Geometry check sheet. Reference: the model listing, model coordinates, mm. A direction names the side the tool comes from. Give positions to 0.01 mm unless a question says otherwise; leave off trailing zeros. Write each loop counter-clockwise with the first axis right and the second up, starting at its lowest first coordinate (ties: lowest second). Pieces come first, ordered by that corner, then holes. Notation, with made-up numbers: (64, 68) -> (76, 68) arc R15 ccw to (76, 88) -> close; hole circle Ø11 at (41, 63.5). An arc over 180 degrees is marked (long way). Write item = value, one per line. Start each with the question number.
1. Set-up check for faces 1 (the flat face through (-0.1, -7.3, -9)), 2 (the flat face through (3, 6, -11)), 3 (the flat face through (-6, 4, -9)): record each of +Z, -Z, +X, -X, +Y, -Y from which the full face is reachable in a straight line by a thin tool's end or side.
2. Mould release check, pull along Z, two halves, no side actions. Record for faces 4 (the flat face through (6, -4, -9)), 5 (the cylindrical face through (-7.25, 2.28, 1.17)), 6 (the flat face through (3, -6, 0)): pulls with the +Z half, pulls with the -Z half, needs draft (parallel to the pull), parting line crosses it, or undercut.
3. Thickness scan on line 1 along Z through (x, y) = (6.75, 2); line 2 along Z through (x, y) = (0.25, 0.75); line 3 along Z through (x, y) = (-0.75, 4.75). Record the ranges inside material, lowest first.
4. Depth check by flat-ended pin: P1, Ø1.5, axis at x = 0.5, z = -12.5, coming from the -Y side; P2, Ø3, axis at x = -6, y = 5, coming from the -Z side; P3, Ø3, axis at y = 6, z = -14.5, coming from the -X side. Enter the tip coordinate at first touch or a pass-through.
5. Cross-section at C-C, the plane z = -3.75. Record the cut outline in (x, y), plus the area to 3 significant figures.
6. Cross-section at A-A, the plane z = -19. Record the cut outline in (x, y), plus the area to 3 significant figures.
```python
from build123d import *

# Parameters (mm, degrees)
BOSS_EXTRUDE1_DEPTH        = 2
SKETCH3_R                  = 6.35
BOSS_EXTRUDE2_DEPTH        = 0.7
SKETCH4_R                  = 6.35
BOSS_EXTRUDE3_DEPTH        = 0.490747729
BOSS_EXTRUDE3_TAPER        = 60.000000001
SKETCH5_R                  = 5.5
BOSS_EXTRUDE4_DEPTH        = 6.309252271
BOSS_EXTRUDE5_DEPTH        = 5
CUT_EXTRUDE1_DEPTH         = 29.154677259
BOSS_EXTRUDE6_DEPTH        = 5
CUT_EXTRUDE2_DEPTH         = 29.330896625
BOSS_EXTRUDE7_DEPTH        = 5
CUT_EXTRUDE3_DEPTH         = 29.311732629
BOSS_EXTRUDE8_DEPTH        = 5
CUT_EXTRUDE4_DEPTH         = 29.498497405
BOSS_EXTRUDE9_REACH        = 28.981
BOSS_EXTRUDE9_START_RADIUS = 6.35
BOSS_EXTRUDE9_END_RADIUS   = 6.35
SKETCH14_W                 = 1
SKETCH14_H                 = 1
FILLET1_R                  = 0.8
SKETCH15_W                 = 5.5
SKETCH15_H                 = 1.6
CUT_EXTRUDE5_DEPTH         = 1


with BuildPart() as part:
    # Sketch1 → Revolve1 (revolve)
    with BuildSketch(Plane.XZ, mode=Mode.PRIVATE) as revolve1_sk:
        Polygon((7.6, 2.3), (0, 2.3), (0, -9), (8, -9), (8, -8.5), (6.35, -8.5), (6.35, 0), (7.6, 0), align=None)
    revolve(revolve1_sk.sketch.rotate(Axis((0, 0, 2.3), (0, 0, -1)), 180), axis=Axis((0, 0, 2.3), (0, 0, -1)))

    # Sketch2 → Boss-Extrude1 (add)
    with BuildSketch(Plane(origin=(0, 0, -9), x_dir=(-1, 0, 0), z_dir=(0, 0, -1))):
        Polygon((-4, -6.92820323), (-8, 0), (-4, 6.92820323), (4, 6.92820323), (8, 0), (4, -6.92820323), align=None)
    extrude(amount=BOSS_EXTRUDE1_DEPTH)

    # Sketch3 → Boss-Extrude2 (add)
    with BuildSketch(Plane(origin=(0, 0, -11), x_dir=(-1, 0, 0), z_dir=(0, 0, -1))):
        Circle(SKETCH3_R)
    extrude(amount=BOSS_EXTRUDE2_DEPTH)

    # Sketch4 → Boss-Extrude3 (add)
    with BuildSketch(Plane(origin=(0, 0, -11.7), x_dir=(-1, 0, 0), z_dir=(0, 0, -1))):
        Circle(SKETCH4_R)
    extrude(amount=BOSS_EXTRUDE3_DEPTH, taper=BOSS_EXTRUDE3_TAPER)

    # Sketch5 → Boss-Extrude4 (add)
    with BuildSketch(Plane(origin=(0, 0, -12.190747729), x_dir=(-1, 0, 0), z_dir=(0, 0, -1))):
        Circle(SKETCH5_R)
    extrude(amount=BOSS_EXTRUDE4_DEPTH)

    # Sketch6 → Boss-Extrude5 (add)
    with BuildSketch(Plane(origin=(0, 0, -18.5), x_dir=(-1, 0, 0), z_dir=(0, 0, -1))):
        Polygon((-4.921641098, -0.547675906), (-4.636324144, -0.454970808), (-4.018290155, -2.357083841), (-4.30360711, -2.449788939), align=None)
    extrude(amount=BOSS_EXTRUDE5_DEPTH)

    # Sketch7 → Cut-Extrude1 (cut, through all)
    with BuildSketch(Plane(origin=(4.327307149, -1.406027324, 0), x_dir=(0, 0, 1), z_dir=(-0.9510565162951721, 0.30901699437489094, 0))):
        with BuildLine():
            Line((-21.4, -0.7), (-20.6, -0.7))
            ThreePointArc((-20.6, -0.7), (-19.9, 0), (-20.6, 0.7))
            Line((-20.6, 0.7), (-21.4, 0.7))
            ThreePointArc((-21.4, 0.7), (-22.1, 0), (-21.4, -0.7))
        make_face()
    extrude(amount=-CUT_EXTRUDE1_DEPTH, mode=Mode.SUBTRACT)

    # Sketch8 → Boss-Extrude6 (add)
    with BuildSketch(Plane(origin=(0, 0, -18.5), x_dir=(-1, 0, 0), z_dir=(0, 0, -1))):
        Polygon((-3.483439892, 3.093242072), (-3.659775468, 3.33594717), (-2.041741479, 4.511517675), (-1.865405904, 4.268812577), align=None)
    extrude(amount=BOSS_EXTRUDE6_DEPTH)

    # Sketch9 → Cut-Extrude2 (cut, through all)
    with BuildSketch(Plane(origin=(2.674422898, 3.681027324, 0), x_dir=(0.8090169943747798, -0.5877852522927041, 0), z_dir=(-0.587785252292704, -0.8090169943747797, 0))):
        with BuildLine():
            Line((0.7, -21.4), (0.7, -20.6))
            ThreePointArc((0.7, -20.6), (0, -19.9), (-0.7, -20.6))
            Line((-0.7, -20.6), (-0.7, -21.4))
            ThreePointArc((-0.7, -21.4), (0, -22.1), (0.7, -21.4))
        make_face()
    extrude(amount=-CUT_EXTRUDE2_DEPTH, mode=Mode.SUBTRACT)

    # Sketch10 → Boss-Extrude7 (add)
    with BuildSketch(Plane(origin=(0, 0, -18.5), x_dir=(-1, 0, 0), z_dir=(0, 0, -1))):
        Polygon((4.636324144, -0.454970808), (4.921641098, -0.547675906), (4.30360711, -2.449788939), (4.018290155, -2.357083841), align=None)
    extrude(amount=BOSS_EXTRUDE7_DEPTH)

    # Sketch11 → Cut-Extrude3 (cut, through all)
    with BuildSketch(Plane(origin=(-4.612624104, -1.498732423, 0), x_dir=(0, 0, 1), z_dir=(-0.9510565162951283, -0.3090169943750252, 0))):
        with BuildLine():
            Line((-20.6, 0.7), (-21.4, 0.7))
            ThreePointArc((-21.4, 0.7), (-22.1, 0), (-21.4, -0.7))
            Line((-21.4, -0.7), (-20.6, -0.7))
            ThreePointArc((-20.6, -0.7), (-19.9, 0), (-20.6, 0.7))
        make_face()
    extrude(amount=-CUT_EXTRUDE3_DEPTH, mode=Mode.SUBTRACT)

    # Sketch12 → Boss-Extrude8 (add)
    with BuildSketch(Plane(origin=(0, 0, -18.5), x_dir=(-1, 0, 0), z_dir=(0, 0, -1))):
        Polygon((1.865405904, 4.268812577), (2.041741479, 4.511517675), (3.659775468, 3.33594717), (3.483439892, 3.093242072), align=None)
    extrude(amount=BOSS_EXTRUDE8_DEPTH)

    # Sketch13 → Cut-Extrude4 (cut, through all)
    with BuildSketch(Plane(origin=(-2.850758474, 3.923732423, 0), x_dir=(-0.8090169943749189, -0.5877852522925126, 0), z_dir=(-0.5877852522925126, 0.8090169943749189, 0))):
        with BuildLine():
            Line((-0.7, -20.6), (-0.7, -21.4))
            ThreePointArc((-0.7, -21.4), (0, -22.1), (0.7, -21.4))
            Line((0.7, -21.4), (0.7, -20.6))
            ThreePointArc((0.7, -20.6), (0, -19.9), (-0.7, -20.6))
        make_face()
    extrude(amount=-CUT_EXTRUDE4_DEPTH, mode=Mode.SUBTRACT)

    # Boss-Extrude9: from a cylinder face, 28.981 long prism both ways, kept between that surface and its translate by the depth
    boss_extrude9_start = Plane(origin=(0, 0, -0.5), z_dir=(0, 0, -1)) * Cylinder(BOSS_EXTRUDE9_START_RADIUS, 71.662, mode=Mode.PRIVATE)
    boss_extrude9_end = Plane(origin=(0, 0.369715646, -0.5), z_dir=(0, 0, -1)) * Cylinder(BOSS_EXTRUDE9_END_RADIUS, 71.662, mode=Mode.PRIVATE)
    # Sketch14 → Boss-Extrude9 (add, from a surface)
    with BuildSketch(Plane(origin=(0, -1.5875, 0), x_dir=(1, 0, 0), z_dir=(0, 1, 0)), mode=Mode.PRIVATE) as boss_extrude9_sk1:
        with Locations((0, 0.5)):
            Rectangle(SKETCH14_W, SKETCH14_H)
    boss_extrude9_tool1 = extrude(boss_extrude9_sk1.sketch, amount=BOSS_EXTRUDE9_REACH, both=True, mode=Mode.PRIVATE)
    add(((boss_extrude9_tool1 - boss_extrude9_start) & boss_extrude9_end).solids().sort_by_distance((0, 6.515142, -0.5))[0])

    # Fillet1
    fillet1_edges = [part.edges().sort_by_distance(p)[0] for p in [
        (-4.160948632, -2.40343639, -23.5),
        (-4.778982621, -0.501323357, -23.5),
        (-3.57160768, 3.214594621, -23.5),
        (-1.953573691, 4.390165126, -23.5),
        (4.160948632, -2.40343639, -23.5),
        (4.778982621, -0.501323357, -23.5),
        (1.953573691, 4.390165126, -23.5),
        (3.57160768, 3.214594621, -23.5),
    ]]
    fillet(fillet1_edges, radius=FILLET1_R)

    # Sketch15 → Cut-Extrude5 (cut)
    with BuildSketch(Plane.XY.offset(2.3)):
        Rectangle(SKETCH15_W, SKETCH15_H)
    extrude(amount=-CUT_EXTRUDE5_DEPTH, mode=Mode.SUBTRACT)


solid = part.part
```
Answers:
q1.face_1 = -Z, +X, -X, -Y
q1.face_2 = -Z
q1.face_3 = -Z, -X, +Y
q2.face_4 = pulls with the -Z half
q2.face_5 = needs draft
q2.face_6 = undercut
q3.line_1 = -11 to -8.5, 0 to 2.3
q3.line_2 = -18.5 to 1.3
q3.line_3 = -18.5 to 2.3
q4.P1 = -6.24
q4.P2 = -11.72
q4.P3 = -3.16
q5.outline = circle Ø12.7 at (0, 0)
q5.area = 127 mm^2
q6.outline = (-4.92, -0.55) -> (-4.3, -2.45) -> (-4.02, -2.36) -> (-4.64, -0.45) -> close; (-3.66, 3.34) -> (-3.48, 3.09) -> (-1.87, 4.27) -> (-2.04, 4.51) -> close; (1.87, 4.27) -> (3.48, 3.09) -> (3.66, 3.34) -> (2.04, 4.51) -> close; (4.02, -2.36) -> (4.3, -2.45) -> (4.92, -0.55) -> (4.64, -0.45) -> close
q6.area = 2.40 mm^2
